For this review, take the finished solid that the model builds, in its own axes (mm). Face numbers are marked on the shaded views. A direction names the side the tool comes from. Coordinates: 2 decimals unless noted, no trailing zeros. Write each loop counter-clockwise with the first axis right and the second up, starting at its lowest first coordinate (ties: lowest second). Pieces come first, ordered by that corner, then holes.
```python
from build123d import *

# Parameters (mm, degrees)
BOSS_EXTRU_1_DEPTH      = 40
ESQUISSE2_R             = 8
ENL_V_MAT_EXTRU_1_DEPTH = 192.268559563
ESQUISSE3_R             = 8
ENL_V_MAT_EXTRU_2_DEPTH = 185.632839971
BOSS_EXTRU_2_DEPTH      = 6.35
BOSS_EXTRU_3_START      = 6.35
BOSS_EXTRU_3_DEPTH      = 6.35
ENL_V_START             = -9.5
ENL_V_MAT_EXTRU_3_DEPTH = 9.5
ENL_V_MAT_EXTRU_4_DEPTH = 9.5


with BuildPart() as part:
    # Esquisse1 → Boss.-Extru.1 (new body)
    with BuildSketch(Plane.XY):
        with BuildLine():
            ThreePointArc((-12.905469818, 18.430920997), (3.907083998, 22.158174443), (18.430920997, 12.905469818))
            Line((18.430920997, 12.905469818), (-30.570908371, 82.887334756))
            Line((-30.570908371, 82.887334756), (-42.858189035, 74.28368821))
            Line((-42.858189035, 74.28368821), (-75.591001848, 121.030989584))
            Line((-75.591001848, 121.030989584), (-81.73464218, 116.729166311))
            Line((-81.73464218, 116.729166311), (-12.905469818, 18.430920997))
        make_face()
        with BuildLine():
            ThreePointArc((-22.5, 0), (-19.957743747, 10.389343798), (-12.905469818, 18.430920997))
            Line((-12.905469818, 18.430920997), (-81.73464218, 116.729166311))
            Line((-81.73464218, 116.729166311), (-87.878282512, 112.427343039))
            Line((-87.878282512, 112.427343039), (-55.1454697, 65.680041665))
            Line((-55.1454697, 65.680041665), (-88.25, 42.5))
            Line((-88.25, 42.5), (-88.25, 7.5))
            Line((-88.25, 7.5), (-140, 7.5))
            Line((-140, 7.5), (-140, 0))
            Line((-140, 0), (-22.5, 0))
        make_face()
        with BuildLine():
            Line((-88.25, -22.560492565), (0.015421683, -22.499994715))
            ThreePointArc((0.015421683, -22.499994715), (-15.904449254, -15.915354031), (-22.5, 0))
            Line((-22.5, 0), (-140, 0))
            Line((-140, 0), (-140, -7.5))
            Line((-140, -7.5), (-88.25, -7.5))
            Line((-88.25, -7.5), (-88.25, -22.560492565))
        make_face()
        with BuildLine():
            ThreePointArc((22.5, 0), (21.458631392, 6.765880489), (18.430920997, 12.905469818))
            ThreePointArc((18.430920997, 12.905469818), (3.907083998, 22.158174443), (-12.905469818, 18.430920997))
            Line((-12.905469818, 18.430920997), (-5.448976145, 7.781944421))
            ThreePointArc((-5.448976145, 7.781944421), (4.386611826, 8.426602915), (9.5, 0))
            ThreePointArc((9.5, 0), (0, -9.5), (-9.5, 0))
            Line((-9.5, 0), (-22.5, 0))
            ThreePointArc((-22.5, 0), (-15.904449254, -15.915354031), (0.015421683, -22.499994715))
            ThreePointArc((0.015421683, -22.499994715), (15.915354031, -15.904449254), (22.5, 0))
        make_face()
        with BuildLine():
            Line((-5.448976145, 7.781944421), (-12.905469818, 18.430920997))
            ThreePointArc((-12.905469818, 18.430920997), (-19.957743747, 10.389343798), (-22.5, 0))
            Line((-22.5, 0), (-9.5, 0))
            ThreePointArc((-9.5, 0), (-8.426602915, 4.386611826), (-5.448976145, 7.781944421))
        make_face()
        with BuildLine():
            ThreePointArc((22.5, 0), (21.458631392, 6.765880489), (18.430920997, 12.905469818))
            ThreePointArc((18.430920997, 12.905469818), (3.907083998, 22.158174443), (-12.905469818, 18.430920997))
            Line((-12.905469818, 18.430920997), (-5.448976145, 7.781944421))
            ThreePointArc((-5.448976145, 7.781944421), (4.386611826, 8.426602915), (9.5, 0))
            ThreePointArc((9.5, 0), (0, -9.5), (-9.5, 0))
            Line((-9.5, 0), (-22.5, 0))
            ThreePointArc((-22.5, 0), (-15.904449254, -15.915354031), (0.015421683, -22.499994715))
            ThreePointArc((0.015421683, -22.499994715), (15.915354031, -15.904449254), (22.5, 0))
        make_face()
        with BuildLine():
            Line((-5.448976145, 7.781944421), (-12.905469818, 18.430920997))
            ThreePointArc((-12.905469818, 18.430920997), (-19.957743747, 10.389343798), (-22.5, 0))
            Line((-22.5, 0), (-9.5, 0))
            ThreePointArc((-9.5, 0), (-8.426602915, 4.386611826), (-5.448976145, 7.781944421))
        make_face()
    extrude(amount=BOSS_EXTRU_1_DEPTH)

    # Esquisse2 → Enlèv. mat.-Extru.1 (cut, through all)
    with BuildSketch(Plane(origin=(6.143640332, 4.301823273, 0), x_dir=(0, 0, -1), z_dir=(0.8191520442889931, 0.5735764363510444, 0))):
        with Locations(Location((-20, 122.5, 0), (0, 0, 90))):
            Circle(ESQUISSE2_R)
        with BuildLine():
            ThreePointArc((-40, 122.5), (-34.142135624, 136.642135624), (-20, 142.5))
            Line((-20, 142.5), (-40, 142.5))
            Line((-40, 142.5), (-40, 122.5))
        make_face()
        with BuildLine():
            ThreePointArc((-20, 142.5), (-5.857864376, 136.642135624), (0, 122.5))
            Line((0, 122.5), (0, 142.5))
            Line((0, 142.5), (-20, 142.5))
        make_face()
    extrude(amount=-ENL_V_MAT_EXTRU_1_DEPTH, mode=Mode.SUBTRACT)

    # Esquisse3 → Enlèv. mat.-Extru.2 (cut, through all)
    with BuildSketch(Plane(origin=(0, 7.5, 0), x_dir=(1, 0, 0), z_dir=(0, 1, 0))):
        with BuildLine():
            ThreePointArc((-140, -20), (-134.142135624, -5.857864376), (-120, 0))
            Line((-120, 0), (-140, 0))
            Line((-140, 0), (-140, -20))
        make_face()
        with BuildLine():
            ThreePointArc((-120, -40), (-134.142135624, -34.142135624), (-140, -20))
            Line((-140, -20), (-140, -40))
            Line((-140, -40), (-120, -40))
        make_face()
        with Locations(Location((-120, -20, 0), (0, 0, 180))):
            Circle(ESQUISSE3_R)
    extrude(amount=-ENL_V_MAT_EXTRU_2_DEPTH, mode=Mode.SUBTRACT)

    # Esquisse4 → Boss.-Extru.2 (add)
    with BuildSketch(Plane.XY.offset(40)):
        with BuildLine():
            ThreePointArc((22.5, 0), (21.458631392, 6.765880489), (18.430920997, 12.905469818))
            ThreePointArc((18.430920997, 12.905469818), (3.907083998, 22.158174443), (-12.905469818, 18.430920997))
            Line((-12.905469818, 18.430920997), (-5.448976145, 7.781944421))
            ThreePointArc((-5.448976145, 7.781944421), (4.386611826, 8.426602915), (9.5, 0))
            ThreePointArc((9.5, 0), (0, -9.5), (-9.5, 0))
            Line((-9.5, 0), (-22.5, 0))
            ThreePointArc((-22.5, 0), (-15.904449254, -15.915354031), (0.015421683, -22.499994715))
            ThreePointArc((0.015421683, -22.499994715), (15.915354031, -15.904449254), (22.5, 0))
        make_face()
        with BuildLine():
            ThreePointArc((22.5, 0), (21.458631392, 6.765880489), (18.430920997, 12.905469818))
            ThreePointArc((18.430920997, 12.905469818), (3.907083998, 22.158174443), (-12.905469818, 18.430920997))
            Line((-12.905469818, 18.430920997), (-5.448976145, 7.781944421))
            ThreePointArc((-5.448976145, 7.781944421), (4.386611826, 8.426602915), (9.5, 0))
            ThreePointArc((9.5, 0), (0, -9.5), (-9.5, 0))
            Line((-9.5, 0), (-22.5, 0))
            ThreePointArc((-22.5, 0), (-15.904449254, -15.915354031), (0.015421683, -22.499994715))
            ThreePointArc((0.015421683, -22.499994715), (15.915354031, -15.904449254), (22.5, 0))
        make_face()
        with BuildLine():
            Line((-5.448976145, 7.781944421), (-12.905469818, 18.430920997))
            ThreePointArc((-12.905469818, 18.430920997), (-19.957743747, 10.389343798), (-22.5, 0))
            Line((-22.5, 0), (-9.5, 0))
            ThreePointArc((-9.5, 0), (-8.426602915, 4.386611826), (-5.448976145, 7.781944421))
        make_face()
    extrude(amount=BOSS_EXTRU_2_DEPTH)

    # Esquisse5 → Boss.-Extru.3 (add)
    with BuildSketch(Plane(origin=(0, 0, 0), x_dir=(-1, 0, 0), z_dir=(0, 0, -1)).offset(BOSS_EXTRU_3_START)):
        with BuildLine():
            ThreePointArc((12.905469818, 18.430920997), (-3.907083998, 22.158174443), (-18.430920997, 12.905469818))
            ThreePointArc((-18.430920997, 12.905469818), (-19.961303045, -10.382503588), (-0.015421683, -22.499994715))
            ThreePointArc((-0.015421683, -22.499994715), (15.904449254, -15.915354031), (22.5, 0))
            Line((22.5, 0), (9.5, 0))
            ThreePointArc((9.5, 0), (-8.426602915, -4.386611826), (5.448976145, 7.781944421))
            Line((5.448976145, 7.781944421), (12.905469818, 18.430920997))
        make_face()
        with BuildLine():
            ThreePointArc((22.5, 0), (19.957743747, 10.389343798), (12.905469818, 18.430920997))
            Line((12.905469818, 18.430920997), (5.448976145, 7.781944421))
            ThreePointArc((5.448976145, 7.781944421), (8.426602915, 4.386611826), (9.5, 0))
            Line((9.5, 0), (22.5, 0))
        make_face()
        with BuildLine():
            ThreePointArc((12.905469818, 18.430920997), (-3.907083998, 22.158174443), (-18.430920997, 12.905469818))
            ThreePointArc((-18.430920997, 12.905469818), (-19.961303045, -10.382503588), (-0.015421683, -22.499994715))
            ThreePointArc((-0.015421683, -22.499994715), (15.904449254, -15.915354031), (22.5, 0))
            Line((22.5, 0), (9.5, 0))
            ThreePointArc((9.5, 0), (-8.426602915, -4.386611826), (5.448976145, 7.781944421))
            Line((5.448976145, 7.781944421), (12.905469818, 18.430920997))
        make_face()
    extrude(amount=-BOSS_EXTRU_3_DEPTH)

    # Esquisse6 → Enlèv. mat.-Extru.3 (cut)
    with BuildSketch(Plane.XY.offset(40).offset(ENL_V_START)):
        with BuildLine():
            Line((18.430920997, 12.905469818), (-25.121932226, 75.105390335))
            Line((-25.121932226, 75.105390335), (-31.265572558, 70.803567062))
            ThreePointArc((-31.265572558, 70.803567062), (-34.349807433, 65.962288063), (-33.107389617, 60.358103458))
            Line((-33.107389617, 60.358103458), (-8.758312615, 25.58401767))
            ThreePointArc((-8.758312615, 25.58401767), (-5.784309245, 23.08853254), (-1.961004212, 22.414380707))
            ThreePointArc((-1.961004212, 22.414380707), (9.508910889, 20.391925208), (18.430920997, 12.905469818))
        make_face()
        with BuildLine():
            Line((-78.75, -22.553981187), (0.015421683, -22.499994715))
            ThreePointArc((0.015421683, -22.499994715), (-11.243321555, -19.489425862), (-19.485571585, -11.25))
            ThreePointArc((-19.485571585, -11.25), (-22.230762114, -8.504809472), (-25.980762114, -7.5))
            Line((-25.980762114, -7.5), (-71.25, -7.5))
            ThreePointArc((-71.25, -7.5), (-76.553300859, -9.696699141), (-78.75, -15))
            Line((-78.75, -15), (-78.75, -22.553981187))
        make_face()
        with BuildLine():
            Line((-22.671091572, 19.301823273), (-45.394670282, 51.754456912))
            ThreePointArc((-45.394670282, 51.754456912), (-50.235949281, 54.838691787), (-55.840133886, 53.596273972))
            Line((-55.840133886, 53.596273972), (-75.551823273, 39.794000473))
            ThreePointArc((-75.551823273, 39.794000473), (-77.902581249, 37.11347474), (-78.75, 33.650360141))
            Line((-78.75, 33.650360141), (-78.75, 15))
            ThreePointArc((-78.75, 15), (-76.553300859, 9.696699141), (-71.25, 7.5))
            Line((-71.25, 7.5), (-28.814731905, 7.5))
            ThreePointArc((-28.814731905, 7.5), (-22.162150656, 11.536885401), (-22.671091572, 19.301823273))
        make_face()
    extrude(amount=ENL_V_MAT_EXTRU_3_DEPTH, mode=Mode.SUBTRACT)

    # Esquisse7 → Enlèv. mat.-Extru.4 (cut)
    with BuildSketch(Plane(origin=(0, 0, 0), x_dir=(-1, 0, 0), z_dir=(0, 0, -1))):
        with BuildLine():
            Line((25.980762114, -7.5), (71.25, -7.5))
            ThreePointArc((71.25, -7.5), (76.553300859, -9.696699141), (78.75, -15))
            Line((78.75, -15), (78.75, -22.553981187))
            Line((78.75, -22.553981187), (-0.015421683, -22.499994715))
            ThreePointArc((-0.015421683, -22.499994715), (11.243321555, -19.489425862), (19.485571585, -11.25))
            ThreePointArc((19.485571585, -11.25), (22.230762114, -8.504809472), (25.980762114, -7.5))
        make_face()
        with BuildLine():
            Line((33.107389617, 60.358103458), (8.758312615, 25.58401767))
            ThreePointArc((8.758312615, 25.58401767), (5.784309245, 23.08853254), (1.961004212, 22.414380707))
            ThreePointArc((1.961004212, 22.414380707), (-9.508910889, 20.391925208), (-18.430920997, 12.905469818))
            Line((-18.430920997, 12.905469818), (25.121932226, 75.105390335))
            Line((25.121932226, 75.105390335), (31.265572558, 70.803567062))
            ThreePointArc((31.265572558, 70.803567062), (34.349807433, 65.962288063), (33.107389617, 60.358103458))
        make_face()
        with BuildLine():
            Line((78.75, 33.650360141), (78.75, 15))
            ThreePointArc((78.75, 15), (76.553300859, 9.696699141), (71.25, 7.5))
            Line((71.25, 7.5), (28.814731905, 7.5))
            ThreePointArc((28.814731905, 7.5), (22.162150656, 11.536885401), (22.671091572, 19.301823273))
            Line((22.671091572, 19.301823273), (45.394670282, 51.754456912))
            ThreePointArc((45.394670282, 51.754456912), (50.235949281, 54.838691787), (55.840133886, 53.596273972))
            Line((55.840133886, 53.596273972), (75.551823273, 39.794000473))
            ThreePointArc((75.551823273, 39.794000473), (77.902581249, 37.11347474), (78.75, 33.650360141))
        make_face()
    extrude(amount=-ENL_V_MAT_EXTRU_4_DEPTH, mode=Mode.SUBTRACT)


solid = part.part
```
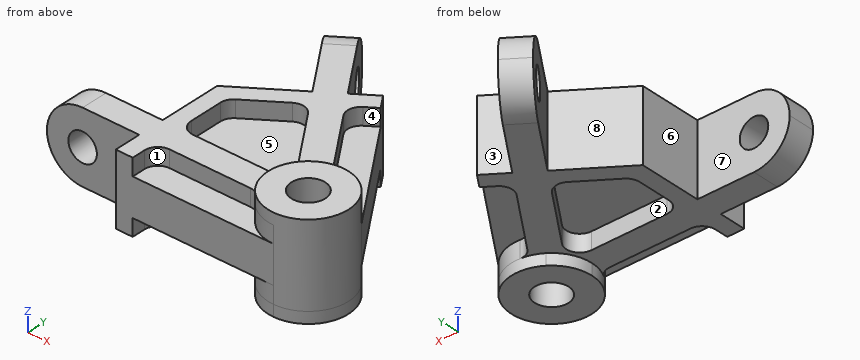
Q1. Draft analysis for pull direction Y (two halves, no side actions). For the marked faces 6, 7 and 8, state which applies: +Y half, -Y half, draft (parallel to the pull), parting line (faces both ways), or undercut.
Ans:
face 6: draft
face 7: +Y half
face 8: undercut
Q2. Add section C-C (x = -38). State the section outline as (y, z) points.
Ans:
outline: (-22.53, 9.5) - (-7.5, 9.5) - (-7.5, 0) - (7.5, 0) - (7.5, 9.5) - (41.19, 9.5) - (41.19, 0) - (77.69, 0) - (77.69, 40) - (41.19, 40) - (41.19, 30.5) - (7.5, 30.5) - (7.5, 40) - (-7.5, 40) - (-7.5, 30.5) - (-22.53, 30.5) - close
Q3. Add section B-B (x = -16). State the section outline as (y, z) points, then the cut area to 3 significant figures.
Ans:
outline: (-22.51, 9.5) - (-15.82, 9.5) - (-15.82, -6.35) - (15.82, -6.35) - (15.82, 0) - (35.93, 0) - (35.93, 9.5) - (62.08, 9.5) - (62.08, 30.5) - (35.93, 30.5) - (35.93, 40) - (15.82, 40) - (15.82, 46.35) - (-15.82, 46.35) - (-15.82, 30.5) - (-22.51, 30.5) - close
area: 3,160 mm2
Q4. Clearance check with flat-ended pins moving along their axes: pin 1 Ø4 at (y, z) = (80, 5) entering from +X; pin 2 Ø7.5 at (x, z) = (-52.5, 34.5) entering from +Y; pin 3 Ø7.5 at (x, z) = (-53.5, 3.5) entering from +Y. State where each tip first meets the part, or that it passes through.
Ans:
pin 1: stops at x = -27.15
pin 2: stops at y = 93.41
pin 3: stops at y = 94.84
Q5. Add section A-A (z = 14.5). State the section outline as (x, y) points.
Ans:
outline: (-139.23, -7.5) - (-125.81, -7.5) - (-125.81, 7.5) - (-139.23, 7.5) - close; (-114.19, -7.5) - (-88.25, -7.5) - (-88.25, -22.56) - (0.02, -22.5) arc R22.5 ccw to (18.43, 12.91) - (-30.57, 82.89) - (-42.86, 74.28) - (-60.79, 99.89) - (-73.07, 91.29) - (-55.15, 65.68) - (-88.25, 42.5) - (-88.25, 7.5) - (-114.19, 7.5) - close; (-87.44, 111.8) - (-79.74, 100.8) - (-67.45, 109.41) - (-75.15, 120.4) - close; hole circle Ø19 at (0, 0)
Q6. For probe 1 along Z at (x, y) = (-120, 1); probe 2 along Y at (x, z) = (-70, 9); probe 3 along Y at (x, z) = (0, 32), list the stretches that pass through material, from the lowest coordinate up.
Ans:
probe 1: z = 0 to 12, 28 to 40
probe 2: y = -7.5 to 7.5, 43.68 to 55.28, 86.89 to 113.05
probe 3: y = -22.5 to -9.5, 9.5 to 22.5
Q7. Tool access review of the marked faces 1, 2, 3, 4 and 5: name each direction out of +Z, -Z, +X, -X, +Y, -Y from which nothing blocks a thin tool from reaching the whole face with its end or side.
Ans:
face 1: +Z, -Y
face 2: -Z
face 3: +Z, -Z, +Y
face 4: +Z, +X
face 5: +Z
